Could you check a few things on this model? Use its own coordinates, in mm. Face numbers are marked on the shaded views. Give positions to 0.01 mm unless a question says otherwise; leave off trailing zeros. Order: outer loops, then holes, each group sorted by start corner. A loop starts at its lowest first (then second) coordinate and runs counter-clockwise, first axis right, second up.
from build123d import *

# Parameters (mm, degrees)
ESBO_O1_R                = 7.5
ESBO_O1_R_2              = 5.5
RESSALTO_EXTRUS_O1_DEPTH = 13
ESBO_O2_W                = 0.5
ESBO_O2_H                = 13
RESSALTO_EXTRUS_O2_DEPTH = 35
ESBO_O3_R                = 2.5
CORTE_EXTRUS_O1_DEPTH    = 20
FILETE1_R                = 5


with BuildPart() as part:
    # Esboço1 → Ressalto-extrusão1 (new body)
    with BuildSketch(Plane.XY):
        Circle(ESBO_O1_R)
        Circle(ESBO_O1_R_2, mode=Mode.SUBTRACT)
    extrude(amount=RESSALTO_EXTRUS_O1_DEPTH)

    # Esboço2 → Ressalto-extrusão2 (add)
    with BuildSketch(Plane(origin=(0, 0, 0), x_dir=(1, 0, 0), z_dir=(0, 1, 0))):
        with Locations((-7.25, -6.5)):
            Rectangle(ESBO_O2_W, ESBO_O2_H)
    extrude(amount=RESSALTO_EXTRUS_O2_DEPTH)

    # Esboço3 → Corte-extrusão1 (cut)
    with BuildSketch(Plane.ZY.offset(7.5)):
        with Locations((6.5, 30)):
            Circle(ESBO_O3_R)
    extrude(amount=-CORTE_EXTRUS_O1_DEPTH, mode=Mode.SUBTRACT)

    # Filete1
    filete1_edges = [part.edges().sort_by_distance(p)[0] for p in [
        (-7.25, 35, 13),
        (-7.25, 35, 0),
    ]]
    fillet(filete1_edges, radius=FILETE1_R)


solid = part.part
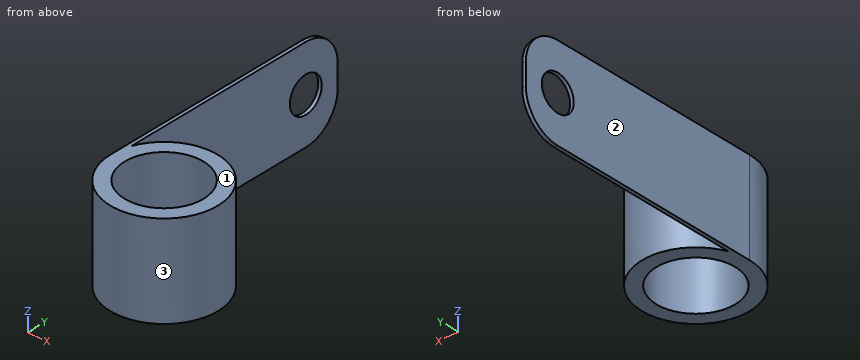
Item 1: Imagine slicing it at C-C on y = -1. List the corners of the cut face in (x, z) for me, then the cut area to 3 significant figures.
Findings:
outline: (-7.43, 0) - (-5.41, 0) - (-5.41, 13) - (-7.43, 13) - close; (5.41, 0) - (7.43, 0) - (7.43, 13) - (5.41, 13) - close
area: 52.6 mm2
Item 2: Please list where these lines run through material, in increasing order: line 1 along X through (y, z) = (5, 7.5); line 2 along Y through (x, z) = (0, 3.75); line 3 along Y through (x, z) = (-3, 9.75).
Findings:
line 1: x = -7.5 to -7, -5.59 to -2.29, 2.29 to 5.59
line 2: y = -7.5 to -5.5, 5.5 to 7.5
line 3: y = -6.87 to -4.61, 4.61 to 6.87
Item 3: For pin 1 (1 mm diameter, centred on x = 3, z = 11, fed in from -Y); pin 2 (3 mm diameter, centred on y = 12, z = 9, fed in from +X); pin 3 (5 mm diameter, centred on y = 6.5, z = 6.5, fed in from +X); pin 4 (4 mm diameter, centred on x = -2, y = 4.5, fed in from -Z), each with a flat end and sliding along its axis, tell me the tip position at first contact or that it passes through.
Findings:
pin 1: stops at y = -7.07
pin 2: stops at x = -7
pin 3: stops at x = 6.34
pin 4: stops at z = 0
Item 4: Imagine slicing it at B-B on x = 0. List the corners of the cut face in (y, z) for me.
Findings:
outline: (-7.5, 0) - (-5.5, 0) - (-5.5, 13) - (-7.5, 13) - close; (5.5, 0) - (7.5, 0) - (7.5, 13) - (5.5, 13) - close
Item 5: We'd pull the mould along X, two halves only. Please class the marked faces 1, 2 and 3: +X half, -X half, draft (parallel to the pull), parting line (faces both ways), or undercut.
Findings:
face 1: draft
face 2: -X half
face 3: undercut
Item 6: Imagine slicing it at D-D on z = 1. List the corners of the cut face in (x, y) for me.
Findings:
outline: (-7.5, 0) arc R7.5 ccw (long way) to (-7, 2.69) - (-7, 33) - (-7.5, 33) - close; hole circle Ø11 at (0, 0)
Item 7: Imagine slicing it at A-A on z = 6.5. List the corners of the cut face in (x, y) for me.
Findings:
outline: (-7.5, 0) arc R7.5 ccw (long way) to (-7, 2.69) - (-7, 27.5) - (-7.5, 27.5) - close; (-7.5, 32.5) - (-7, 32.5) - (-7, 35) - (-7.5, 35) - close; hole circle Ø11 at (0, 0)
